The listing builds one solid part. Answer for the finished solid, in the listing's coordinates (mm). A direction names the side the tool comes from. Round coordinates to 2 decimals unless told otherwise and drop trailing zeros. Write each loop counter-clockwise with the first axis right and the second up, starting at its lowest first coordinate (ties: lowest second). Pieces come first, ordered by that corner, then holes. Notation, with made-up numbers: (-20, 45.25) - (-13, 45.25) arc R27 ccw to (-13, 84.25) - close; hole circle Ø4 at (65, -31). An arc over 180 degrees is marked (long way). Return JSON: item names as keys, results as strings. Group by question number.
(1) Section A-A, the plane z = 7 is taken. Give the number of separate pieces and of enclosed holes in the cut face, then the cut area to 3 significant figures.
(2) Each of these flat-tipped pins is pushed along its axis until it touches: pin 1 (9 mm diameter, centred on x = 13, z = 8, fed in from -Y); pin 2 (6 mm diameter, centred on y = 12, z = 19, fed in from +X); pin 3 (2 mm diameter, centred on x = 4.5, z = 9.5, fed in from +Y); pin 4 (6 mm diameter, centred on y = 16, z = 24, fed in from +X). Where does it stop, or does it pass through?
(3) Determine the mould class of faces 1 (the flat face through (3, 12, 17)), 2 (the flat face through (-49, 24, -3)), 3 (the cylindrical face through (8, 26, 7)), 4 (the flat face through (-59, 23, 0)) for opening direction Z: +Z half, -Z half, draft (parallel to the pull), parting line (faces both ways), or undercut.
(4) Which of the six approach directions +Z, -Z, +X, -X, +Y, -Y give full straight-line access (tool end or side, diameter ignored) to faces 5 (the flat face through (-110.5, 16, -1)), 6 (the flat face through (-59, 0, 20)), 7 (the flat face through (3, 1, 17)), 8 (the flat face through (15, 23.75, 9)), 9 (the cylindrical face through (22.6, 20.5, 17.3))?
(5) Section D-D, the plane x = 13 is taken. Write down the section's boundary in (y, z), then the cut area to 3 significant figures.
(6) Find the intervals of material crossed by line 1 along Z through (x, y) = (13, 21); line 2 along Y through (x, z) = (-6, 4.5); line 3 along X through (y, z) = (25, 27), in increasing order. Write a range as [from, to].
(7) Section C-C, the plane z = 15 is taken. Write down the section's boundary in (x, y).
(8) Section B-B, the plane x = -71.5 is taken. Write down the section's boundary in (y, z).
```python
from build123d import *

# Parameters (mm, degrees)
SKETCH1_W                      = 115.5
SKETCH1_H                      = 30.5
SKETCH1_W_2                    = 88
SKETCH1_H_2                    = 12
BOSS_EXTRUDE1_DEPTH            = 3
BOSS_EXTRUDE2_START            = 37
SKETCH1_3_W                    = 115.5
SKETCH1_3_H                    = 30.5
BOSS_EXTRUDE2_DEPTH            = 37
CBORE_FOR_M5_SHCS1_D           = 5.3
CBORE_FOR_M5_SHCS1_CBORE_D     = 10
CBORE_FOR_M5_SHCS1_CBORE_DEPTH = 9.75
FILLET1_R                      = 2


with BuildPart() as part:
    # Sketch1 → Boss-Extrude1 (new body)
    # profile 1 of 2: a face of its own
    with BuildSketch(Plane.XY):
        with BuildLine():
            Line((23, 17), (23, 19))
            ThreePointArc((23, 19), (22.596751829, 20.502291563), (21.495413373, 21.600718909))
            Line((21.495413373, 21.600718909), (1.495413373, 33.100718909))
            ThreePointArc((1.495413373, 33.100718909), (0.773900275, 33.398461379), (0, 33.5))
            Line((0, 33.5), (-118.5, 33.5))
            Line((-118.5, 33.5), (-118.5, -3))
            Line((-118.5, -3), (3, -3))
            Line((3, -3), (3, 4.6))
            Line((3, 4.6), (5, 4.6))
            Line((5, 4.6), (5, 9.4))
            Line((5, 9.4), (3, 9.4))
            Line((3, 9.4), (3, 17))
            Line((3, 17), (23, 17))
        make_face()
        with Locations((-57.75, 15.25)):
            Rectangle(SKETCH1_W, SKETCH1_H, mode=Mode.SUBTRACT)
    # profile 2 of 2: a face of its own
    with BuildSketch(Plane.XY):
        with Locations((-57.75, 15.25)):
            Rectangle(SKETCH1_W, SKETCH1_H)
        with Locations((-66.5, 16)):
            Rectangle(SKETCH1_W_2, SKETCH1_H_2, mode=Mode.SUBTRACT)
    extrude(amount=-BOSS_EXTRUDE1_DEPTH)

    # Sketch1<3> → Boss-Extrude2 (add)
    with BuildSketch(Plane.XY.offset(BOSS_EXTRUDE2_START)):
        with BuildLine():
            Line((23, 17), (23, 19))
            ThreePointArc((23, 19), (22.596751829, 20.502291563), (21.495413373, 21.600718909))
            Line((21.495413373, 21.600718909), (1.495413373, 33.100718909))
            ThreePointArc((1.495413373, 33.100718909), (0.773900275, 33.398461379), (0, 33.5))
            Line((0, 33.5), (-118.5, 33.5))
            Line((-118.5, 33.5), (-118.5, -3))
            Line((-118.5, -3), (3, -3))
            Line((3, -3), (3, 4.6))
            Line((3, 4.6), (5, 4.6))
            Line((5, 4.6), (5, 9.4))
            Line((5, 9.4), (3, 9.4))
            Line((3, 9.4), (3, 17))
            Line((3, 17), (23, 17))
        make_face()
        with Locations((-57.75, 15.25)):
            Rectangle(SKETCH1_3_W, SKETCH1_3_H, mode=Mode.SUBTRACT)
    extrude(amount=-BOSS_EXTRUDE2_DEPTH)

    # CBORE for M5 SHCS1 (through all)
    with Locations(Plane(origin=(0, 33.5, 0), x_dir=(1, 0, 0), z_dir=(0, 1, 0))):
        with Locations((13, -27), (13, -7)):
            CounterBoreHole(CBORE_FOR_M5_SHCS1_D / 2, CBORE_FOR_M5_SHCS1_CBORE_D / 2, CBORE_FOR_M5_SHCS1_CBORE_DEPTH)

    # Fillet1
    fillet1_edges = [part.edges().sort_by_distance(p)[0] for p in [
        (-22.5, 22, -1.5),
        (-110.5, 22, -1.5),
        (-110.5, 10, -1.5),
        (-22.5, 10, -1.5),
        (3, 17, 17),
        (-118.5, -3, 17),
        (-118.5, 33.5, 17),
        (0, 0, 18.5),
        (-57.75, 0, 0),
        (-115.5, 0, 18.5),
    ]]
    fillet(fillet1_edges, radius=FILLET1_R)


solid = part.part
```
Working result:
{
 "1": {"separate pieces": "2", "enclosed holes": "1", "area": "1,050 mm^2"},
 "2": {"pin 1": "stops at y = 17", "pin 2": "stops at x = 5", "pin 3": "stops at y = 31.95", "pin 4": "stops at x = 23"},
 "3": {"face 1": "draft", "face 2": "-Z half", "face 3": "undercut", "face 4": "+Z half"},
 "4": {"face 5": "+Z, -Z", "face 6": "+Z", "face 7": "+Z, -Z, +X, -Y", "face 8": "+Y", "face 9": "+Z, -Z, +X, +Y"},
 "5": {"outline": "(17, -3) - (26.49, -3) - (26.49, 2) - (23.75, 2) - (23.75, 4.35) - (17, 4.35) - close; (17, 9.65) - (23.75, 9.65) - (23.75, 12) - (26.49, 12) - (26.49, 22) - (23.75, 22) - (23.75, 24.35) - (17, 24.35) - close; (17, 29.65) - (23.75, 29.65) - (23.75, 32) - (26.49, 32) - (26.49, 37) - (17, 37) - close", "area": "253 mm^2"},
 "6": {"line 1": "z = [-3, 4.35], [9.65, 24.35], [29.65, 37]", "line 2": "y = [-3, 0], [30.5, 33.5]", "line 3": "x = [-118.5, -115.5], [0, 8]"},
 "7": {"outline": "(-118.5, -1) arc R2 ccw to (-116.5, -3) - (3, -3) - (3, 4.6) - (5, 4.6) - (5, 9.4) - (3, 9.4) - (3, 15) arc R2 cw to (5, 17) - (23, 17) - (23, 19) arc R3 ccw to (21.5, 21.6) - (1.5, 33.1) arc R3 ccw to (0, 33.5) - (-116.5, 33.5) arc R2 ccw to (-118.5, 31.5) - close; hole (-115.5, 2) arc R2 ccw to (-113.5, 0) - (-2, 0) arc R2 ccw to (0, 2) - (0, 30.5) - (-115.5, 30.5) - close"},
 "8": {"outline": "(-3, -3) - (10, -3) - (10, 0) - (2, 0) arc R2 cw to (0, 2) - (0, 37) - (-3, 37) - close; (22, -3) - (33.5, -3) - (33.5, 37) - (30.5, 37) - (30.5, 0) - (22, 0) - close"}
}
